Design review of the part built by this model. Coordinates are the model's own, in mm. A direction names the side the tool comes from. Coordinates: 2 decimals unless noted, no trailing zeros. Order: outer loops, then holes, each group sorted by start corner. A loop starts at its lowest first (then second) coordinate and runs counter-clockwise, first axis right, second up. Notation, with made-up numbers: (81, 26) -> (140, 26) arc R19 cw to (140, 37) -> close; hole circle Ø5 at (14, -5). An arc over 180 degrees is marked (long way). Write item = value, one per line.
```python
from build123d import *

# Parameters (mm, degrees)
ESTRUSIONE_ESTRUSIONE1_DEPTH = 6.4


with BuildPart() as part:
    # Schizzo1 → Estrusione-Estrusione1 (new body)
    with BuildSketch(Plane.XY):
        with BuildLine():
            Line((0, -34), (0, -2))
            ThreePointArc((0, -2), (-0.585786438, -0.585786438), (-2, 0))
            Line((-2, 0), (-40, 0))
            Line((-40, 0), (-98, 0))
            Line((-98, 0), (-136, 0))
            ThreePointArc((-136, 0), (-137.414213562, -0.585786438), (-138, -2))
            Line((-138, -2), (-138, -34))
            ThreePointArc((-138, -34), (-137.414213562, -35.414213562), (-136, -36))
            Line((-136, -36), (-98, -36))
            Line((-98, -36), (-40, -36))
            Line((-40, -36), (-2, -36))
            ThreePointArc((-2, -36), (-0.585786438, -35.414213562), (0, -34))
        make_face()
        with BuildLine():
            Line((-19.5, -24.5), (-13.5, -24.5))
            ThreePointArc((-13.5, -24.5), (-7, -18), (-13.5, -11.5))
            Line((-13.5, -11.5), (-19.5, -11.5))
            ThreePointArc((-19.5, -11.5), (-26, -18), (-19.5, -24.5))
        make_face(mode=Mode.SUBTRACT)
        with BuildLine():
            Line((-124.5, -24.5), (-118.5, -24.5))
            ThreePointArc((-118.5, -24.5), (-112, -18), (-118.5, -11.5))
            Line((-118.5, -11.5), (-124.5, -11.5))
            ThreePointArc((-124.5, -11.5), (-131, -18), (-124.5, -24.5))
        make_face(mode=Mode.SUBTRACT)
    extrude(amount=ESTRUSIONE_ESTRUSIONE1_DEPTH)


solid = part.part
```
(1) For L1, parallel to Y at x = -121, z = 3.5; L2, parallel to X at y = -15, z = 0.5; L3, parallel to X at y = -12, z = 5.5, list the stretches that pass through material, from the lowest coordinate up.
Report:
L1 = -36 to -24.5, -11.5 to 0
L2 = -138 to -130.27, -112.73 to -25.27, -7.73 to 0
L3 = -138 to -127, -116 to -22, -11 to 0
(2) We need section A-A (z = 1). Write out the cut boundary in (x, y), and give its area (3 significant figures).
Report:
outline = (-138, -34) arc R2 ccw to (-136, -36) -> (-2, -36) arc R2 ccw to (0, -34) -> (0, -2) arc R2 ccw to (-2, 0) -> (-136, 0) arc R2 ccw to (-138, -2) -> close; hole (-124.5, -24.5) -> (-118.5, -24.5) arc R6.5 ccw to (-118.5, -11.5) -> (-124.5, -11.5) arc R6.5 ccw to start; hole (-19.5, -24.5) -> (-13.5, -24.5) arc R6.5 ccw to (-13.5, -11.5) -> (-19.5, -11.5) arc R6.5 ccw to start
area = 4,540 mm²
(3) We need section B-B (y = -15). Write out the cut boundary in (x, z), and give its area (3 significant figures).
Report:
outline = (-138, 0) -> (-130.27, 0) -> (-130.27, 6.4) -> (-138, 6.4) -> close; (-112.73, 0) -> (-25.27, 0) -> (-25.27, 6.4) -> (-112.73, 6.4) -> close; (-7.73, 0) -> (0, 0) -> (0, 6.4) -> (-7.73, 6.4) -> close
area = 659 mm²
(4) For faces 5 (the flat face through (-121, -11.5, 3)), 6 (the flat face through (-70, -18, 0)), list the 3-axis set-ups (+Z, -Z, +X, -X, +Y, -Y) from which the entire face can be reached by the end or side of a thin tool; tool diameter is ignored.
Report:
face_5 = +Z, -Z
face_6 = -Z, +X, -X, +Y, -Y
(5) We need section C-C (y = -22). Write out the cut boundary in (x, z), and give its area (3 significant figures).
Report:
outline = (-138, 0) -> (-129.62, 0) -> (-129.62, 6.4) -> (-138, 6.4) -> close; (-113.38, 0) -> (-24.62, 0) -> (-24.62, 6.4) -> (-113.38, 6.4) -> close; (-8.38, 0) -> (0, 0) -> (0, 6.4) -> (-8.38, 6.4) -> close
area = 675 mm²
(6) The part is to be moulded in two halves that separate along Y. For faces 1 (the flat face through (-70, -18, 6.4)), 2 (the cylindrical face through (-7, -18, 3)), 3 (the flat face through (-70, -36, 3)), 4 (the cylindrical face through (-131, -18, 3)), say which applies: released by +Y, released by -Y, zero draft, split by the parting line, or undercut.
Report:
face_1 = zero draft
face_2 = undercut
face_3 = released by -Y
face_4 = undercut
